```python
from build123d import *

# Parameters (mm, degrees)
SKETCH1_R           = 13.35
SKETCH1_R_2         = 12.6
SKETCH1_R_3         = 1.575
BOSS_EXTRUDE1_DEPTH = 1
SKETCH1_3_R         = 12.6
SKETCH1_3_R_2       = 1.575
BOSS_EXTRUDE2_DEPTH = 6
SKETCH2_R           = 3
CUT_EXTRUDE1_DEPTH  = 3.5
SKETCH3_R           = 2
BOSS_EXTRUDE3_DEPTH = 12


with BuildPart() as part:
    # Sketch1 → Boss-Extrude1 (new body)
    # profile 1 of 2: a face of its own
    with BuildSketch(Plane(origin=(0, 33, 0), x_dir=(1, 0, 0), z_dir=(0, 1, 0))):
        with Locations(Location((0, 0, 0), (0, 0, 270))):
            Circle(SKETCH1_R)
        Circle(SKETCH1_R_2, mode=Mode.SUBTRACT)
    # profile 2 of 2: a face of its own
    with BuildSketch(Plane(origin=(0, 33, 0), x_dir=(1, 0, 0), z_dir=(0, 1, 0))):
        Circle(SKETCH1_R_2)
        with Locations(Location((6, -6, 0), (0, 0, 270))):
            Circle(SKETCH1_R_3, mode=Mode.SUBTRACT)
        with Locations(Location((-6, 6, 0), (0, 0, 270))):
            Circle(SKETCH1_R_3, mode=Mode.SUBTRACT)
        with Locations(Location((6, 6, 0), (0, 0, 270))):
            Circle(SKETCH1_R_3, mode=Mode.SUBTRACT)
        with Locations(Location((-6, -6, 0), (0, 0, 270))):
            Circle(SKETCH1_R_3, mode=Mode.SUBTRACT)
    extrude(amount=BOSS_EXTRUDE1_DEPTH)

    # Sketch1_3 → Boss-Extrude2 (add)
    with BuildSketch(Plane(origin=(0, 33, 0), x_dir=(1, 0, 0), z_dir=(0, 1, 0))):
        with Locations(Location((0, 0, 0), (0, 0, 270))):
            Circle(SKETCH1_3_R)
        with Locations(Location((6, -6, 0), (0, 0, 270))):
            Circle(SKETCH1_3_R_2, mode=Mode.SUBTRACT)
        with Locations(Location((-6, 6, 0), (0, 0, 270))):
            Circle(SKETCH1_3_R_2, mode=Mode.SUBTRACT)
        with Locations(Location((6, 6, 0), (0, 0, 270))):
            Circle(SKETCH1_3_R_2, mode=Mode.SUBTRACT)
        with Locations(Location((-6, -6, 0), (0, 0, 270))):
            Circle(SKETCH1_3_R_2, mode=Mode.SUBTRACT)
    extrude(amount=BOSS_EXTRUDE2_DEPTH)

    # Sketch2 → Cut-Extrude1 (cut)
    with BuildSketch(Plane(origin=(0, 39, 0), x_dir=(1, 0, 0), z_dir=(0, 1, 0))):
        with Locations(Location((-6, 6, 0), (0, 0, 270))):
            Circle(SKETCH2_R)
        with Locations(Location((6, 6, 0), (0, 0, 270))):
            Circle(SKETCH2_R)
        with Locations(Location((6, -6, 0), (0, 0, 270))):
            Circle(SKETCH2_R)
        with Locations(Location((-6, -6, 0), (0, 0, 270))):
            Circle(SKETCH2_R)
    extrude(amount=-CUT_EXTRUDE1_DEPTH, mode=Mode.SUBTRACT)

    # Sketch3 → Boss-Extrude3 (add)
    with BuildSketch(Plane(origin=(0, 39, 0), x_dir=(1, 0, 0), z_dir=(0, 1, 0))):
        with Locations(Location((0, 0, 0), (0, 0, 270))):
            Circle(SKETCH3_R)
    extrude(amount=BOSS_EXTRUDE3_DEPTH)


solid = part.part
```
Check sheet for the modelled part. Datum: model origin and axes. Units: mm. A direction names the side the tool comes from. Round coordinates to 2 decimals unless told otherwise and drop trailing zeros. Loops run counter-clockwise (first coordinate to the right, second up) from the corner with the lowest first, then second, coordinate; pieces in that order, holes last. Notation, with made-up numbers: (47, 50) -> (60, 50) arc R26 ccw to (60, 72) -> close; hole circle Ø9 at (-34, 38). An arc over 180 degrees is marked (long way). Answer in a Markdown table with one row per item.
Q1. Thickness scan on L1, parallel to Z at x = 6, y = 33.6 (3 decimals); L2, parallel to X at y = 37.65, z = 6; L3, parallel to Y at x = 5, z = -0.75. Record the ranges inside material, lowest first.
Data:
| item | result |
|---|---|
| L1 | z = -11.926 to -7.575, -4.425 to 4.425, 7.575 to 11.926 |
| L2 | x = -11.08 to -9, -3 to 3, 9 to 11.08 |
| L3 | y = 33 to 39 |
Q2. Release check for a two-part mould opening along X. For faces 1 (the face through (-8, 34, 10)), 2 (the face through (3.338, 37.274, -4.616)), 3 (the face through (3.338, 37.274, 7.384)), 4 (the face through (-5.113, 33.493, 12.332)) record: released by +X, released by -X, zero draft, split by the parting line, or undercut.
Data:
| item | result |
|---|---|
| face 1 | zero draft |
| face 2 | undercut |
| face 3 | undercut |
| face 4 | split by the parting line |
Q3. Sectioned sample at B-B on x = 0. Enter the section's corners in (y, z).
Data:
| item | result |
|---|---|
| outline | (33, -13.35) -> (34, -13.35) -> (34, -12.6) -> (39, -12.6) -> (39, -2) -> (51, -2) -> (51, 2) -> (39, 2) -> (39, 12.6) -> (34, 12.6) -> (34, 13.35) -> (33, 13.35) -> close |
Q4. Sectioned sample at D-D on z = -0.25. Enter the section's corners in (x, y).
Data:
| item | result |
|---|---|
| outline | (-13.35, 33) -> (13.35, 33) -> (13.35, 34) -> (12.6, 34) -> (12.6, 39) -> (1.98, 39) -> (1.98, 51) -> (-1.98, 51) -> (-1.98, 39) -> (-12.6, 39) -> (-12.6, 34) -> (-13.35, 34) -> close |
Q5. Go/stop test with flat-tipped pins: P1, Ø6.5, axis at x = 4.5, z = -6.5, coming from the +Y side; P2, Ø5, axis at y = 45.5, z = -3, coming from the -X side; P3, Ø1.9, axis at x = 6, z = 6, coming from the +Y side; P4, Ø3.5, axis at x = 6, z = -6, coming from the +Y side. Record where each tip stops, or that it passes through.
Data:
| item | result |
|---|---|
| P1 | stops at y = 39 |
| P2 | stops at x = -1.94 |
| P3 | passes through |
| P4 | stops at y = 35.5 |
Q6. Set-up check for faces 5 (the face through (-7.3, 35.5, -4.7)), 6 (the face through (-4.936, 34.232, -7.161)): record each of +Z, -Z, +X, -X, +Y, -Y from which the full face is reachable in a straight line by a thin tool's end or side.
Data:
| item | result |
|---|---|
| face 5 | +Y |
| face 6 | +Y, -Y |
Q7. Sectioned sample at C-C on x = -6. Enter the section's corners in (y, z) (3 decimals).
Data:
| item | result |
|---|---|
| outline | (33, -11.926) -> (34, -11.926) -> (34, -11.08) -> (39, -11.08) -> (39, -9) -> (35.5, -9) -> (35.5, -7.575) -> (33, -7.575) -> close; (33, -4.425) -> (35.5, -4.425) -> (35.5, -3) -> (39, -3) -> (39, 3) -> (35.5, 3) -> (35.5, 4.425) -> (33, 4.425) -> close; (33, 7.575) -> (35.5, 7.575) -> (35.5, 9) -> (39, 9) -> (39, 11.08) -> (34, 11.08) -> (34, 11.926) -> (33, 11.926) -> close |
Q8. Sectioned sample at A-A on z = -6. Enter the section's corners in (x, y) (3 decimals).
Data:
| item | result |
|---|---|
| outline | (-11.926, 33) -> (-7.575, 33) -> (-7.575, 35.5) -> (-9, 35.5) -> (-9, 39) -> (-11.08, 39) -> (-11.08, 34) -> (-11.926, 34) -> close; (-4.425, 33) -> (4.425, 33) -> (4.425, 35.5) -> (3, 35.5) -> (3, 39) -> (-3, 39) -> (-3, 35.5) -> (-4.425, 35.5) -> close; (7.575, 33) -> (11.926, 33) -> (11.926, 34) -> (11.08, 34) -> (11.08, 39) -> (9, 39) -> (9, 35.5) -> (7.575, 35.5) -> close |
